Geometry: final body of the model. Coordinates: model frame, mm. Coordinates: 2 decimals unless noted, no trailing zeros. Order: outer loops, then holes, each group sorted by start corner. A loop starts at its lowest first (then second) coordinate and runs counter-clockwise, first axis right, second up. Notation, with made-up numbers: (8.5, 3) -> (52.5, 3) arc R31 cw to (52.5, 31) -> close; hole circle Ø1 at (-21, 68.25). An arc over 180 degrees is marked (long way). Answer in a Markdown table with one row per item. Add a question column.
1) Section query B-B on x = 0. Return the cut outline in (y, z) (1 decimal), then the cut area to 3 significant figures.
2) Contact query for flat-ended pins moving along their axis: P1, Ø1.5, axis at y = -1.5, z = 1.5, coming from the -X side; P2, Ø3, axis at x = 0, y = 10, coming from the +Z side. Output: stop coordinate, or through.
3) Ray query, line 1 (Y direction, x = 1, z = 2.3); line 2 (X direction, y = -2.5, z = 2.5); line 3 (X direction, y = -2.75, z = 0.3). Return the intervals inside material, ascending. Write a range as from..to.
4) Section query A-A on y = 0. Return the cut outline in (x, z) (3 decimals).
5) Section query C-C on x = -2. Return the cut outline in (y, z) (3 decimals).
6) Section query D-D on z = 1.9. Count the separate pieces of the cut face and the enclosed holes in it, then the cut area to 3 significant figures.
Autodesk Inventor part; units mm, degrees
ref_plane "YZ Plane" through (0, 0, 0) normal (1, 0, 0) x (0, 1, 0)
ref_plane "XZ Plane" through (0, 0, 0) normal (0, 1, 0) x (-1, 0, 0)
ref_plane "XY Plane" through (0, 0, 0) normal (0, 0, 1) x (1, 0, 0)
sketch "Sketch1" plane through (0, 0, 0) normal (0, 0, 1) x (1, 0, 0)
  circle A0 centre (0, 0) radius 3.175
  circle A1 centre (0, 0) radius 3.81
  circle A2 centre (0, 10) radius 1.5875
  circle A3 centre (0, 10) radius 2.3813
  line L0 (-2.3568, 10.3402) -> (-3.7709, 0.5444)
  line L1 (2.3568, 10.3402) -> (3.7709, 0.5444)
  dimension "d0" = 6.35
  dimension "d1" = 7.62
  dimension "d2" = 3.175
  dimension "d3" = 4.7625
  dimension "d6" = 10
extrude "Extrusion1" add sketch "Sketch1" along normal blind 3.175
Result:
| question | item | result |
|---|---|---|
| 1 | outline | (-3.8, 0) -> (-3.2, 0) -> (-3.2, 3.2) -> (-3.8, 3.2) -> close; (3.2, 0) -> (8.4, 0) -> (8.4, 3.2) -> (3.2, 3.2) -> close; (11.6, 0) -> (12.4, 0) -> (12.4, 3.2) -> (11.6, 3.2) -> close |
| 1 | area | 21.2 mm2 |
| 2 | P1 | x = -3.74 |
| 2 | P2 | through |
| 3 | line 1 | -3.68..-3.01, 3.01..8.77, 11.23..12.16 |
| 3 | line 2 | -2.88..-1.96, 1.96..2.88 |
| 3 | line 3 | -2.64..-1.59, 1.59..2.64 |
| 4 | outline | (-3.81, 0) -> (-3.175, 0) -> (-3.175, 3.175) -> (-3.81, 3.175) -> close; (3.175, 0) -> (3.81, 0) -> (3.81, 3.175) -> (3.175, 3.175) -> close |
| 5 | outline | (-3.243, 0) -> (-2.466, 0) -> (-2.466, 3.175) -> (-3.243, 3.175) -> close; (2.466, 0) -> (11.293, 0) -> (11.293, 3.175) -> (2.466, 3.175) -> close |
| 6 | separate pieces | 1 |
| 6 | enclosed holes | 2 |
| 6 | area | 54.7 mm2 |
